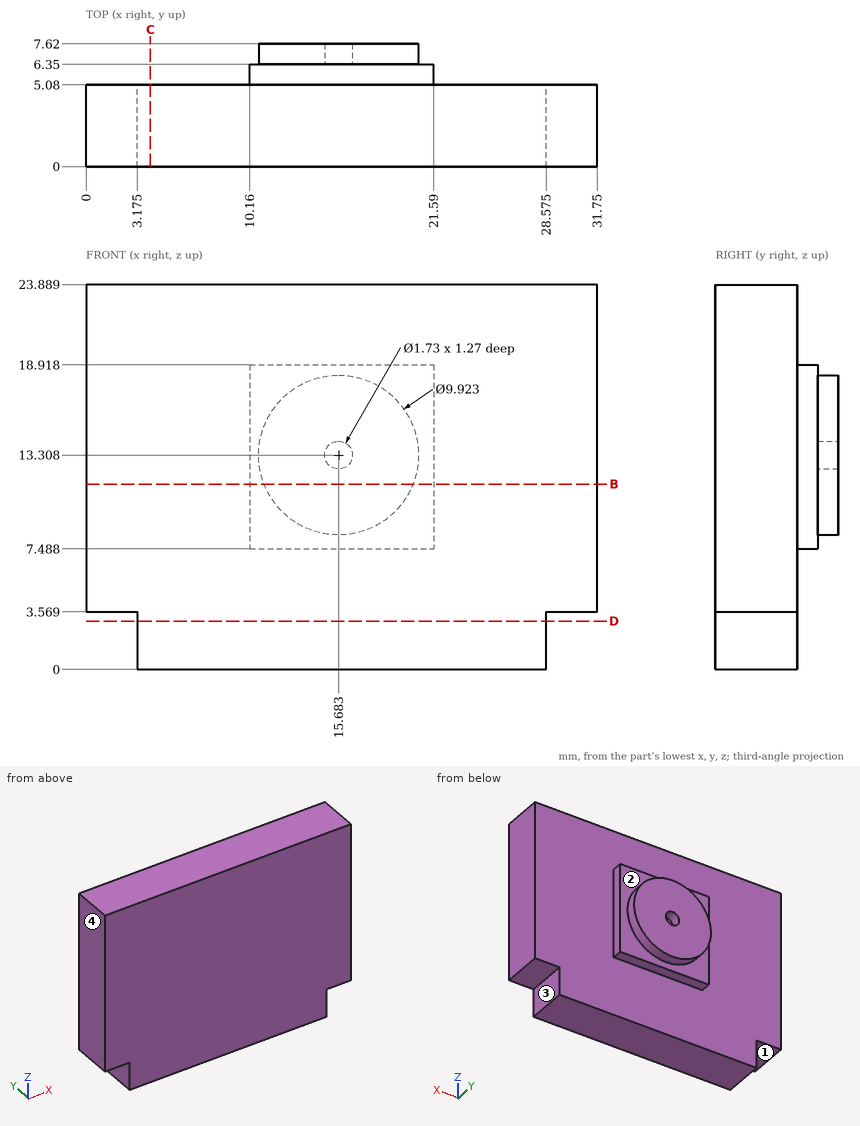
Part print with two shaded views. Sizes in mm from the minimum x, y, z corner. A direction names the side the tool comes from. Give positions to 0.01 mm unless a question says otherwise; leave off trailing zeros. Order: outer loops, then holes, each group sorted by start corner. A loop starts at its lowest first (then second) coordinate and runs counter-clockwise, first axis right, second up. Notation, with made-up numbers: M -23.5,14 L 24.5,14 A14 cw 24.5,19 Z; hole C -10,49.25 d2. An arc over 180 degrees is marked long. Put each result on its own line as item: value.
Item 1: Cut at B-B on z = 11.5. Write the cut outline in (x, y).
Results are:
outline: M 0,0 L 31.75,0 L 31.75,5.08 L 21.59,5.08 L 21.59,6.35 L 20.3,6.35 L 20.3,7.62 L 11.06,7.62 L 11.06,6.35 L 10.16,6.35 L 10.16,5.08 L 0,5.08 Z
Item 2: Drop flat-ended pins along their axis: pin 1 Ø4 at (x, z) = (21, 5) entering from -Y; pin 2 Ø1.6 at (x, y) = (1.5, 1.5) entering from -Z; pin 3 Ø0.6 at (x, y) = (15, 5.5) entering from +Z; pin 4 Ø0.6 at (y, z) = (5.5, 15) entering from +X. Give the stop position or say it passes through.
Results are:
pin 1: y = 0
pin 2: z = 3.57
pin 3: z = 18.92
pin 4: x = 21.59
Item 3: Cut at D-D on z = 3. Write the cut outline in (x, y) (1 decimal), then the cut area to 3 significant figures.
Results are:
outline: M 3.2,0 L 28.6,0 L 28.6,5.1 L 3.2,5.1 Z
area: 129 mm2
Item 4: Cut at C-C on x = 4. Write the cut outline in (y, z), then the cut area to 3 significant figures.
Results are:
outline: M 0,0 L 5.08,0 L 5.08,23.89 L 0,23.89 Z
area: 121 mm2
Item 5: Which spindle directions (+Z, -Z, +X, -X, +Y, -Y) get a long thin tool onto all of the face, cutting with end or side? Do the marked faces 1, 2, 3 and 4. Say none if no direction does.
Results are:
face 1: -Z, -X, +Y, -Y
face 2: +Y
face 3: -Z, +X, +Y, -Y
face 4: +Z, -Z, -X, +Y, -Y
Item 6: Wall check: probe 1 along Y at (x, z) = (9, 3.25); probe 2 along X at (y, z) = (6, 16); probe 3 along Z at (x, y) = (12, 6). Give the ranges that are in metal, low to high.
Results are:
probe 1: 0 to 5.08
probe 2: 10.16 to 21.59
probe 3: 7.49 to 18.92
